Could you check a few things on this model? Use its own coordinates, in mm. Face numbers are marked on the shaded views. A direction names the side the tool comes from. Give positions to 0.01 mm unless a question says otherwise; leave off trailing zeros. Loops run counter-clockwise (first coordinate to the right, second up) from the corner with the lowest first, then second, coordinate; pieces in that order, holes last. Notation, with made-up numbers: (-10, -14) - (14, -14) arc R20 cw to (14, 13) - close; hole circle Ø1 at (76.25, -3.5). An arc over 180 degrees is marked (long way). Answer in a Markdown table with one row per item. Add a question column.
```python
from build123d import *

# Parameters (mm, degrees)
SKETCH_2_W          = 56
SKETCH_2_H          = 30
EXTRUDE_2_DEPTH     = 12
CUT_EXTRUDE_1_DEPTH = 65.652919501
SKETCH_6_W          = 24
SKETCH_6_H          = 30
CUT_EXTRUDE_2_DEPTH = 4
SKETCH_8_W          = 10
SKETCH_8_H          = 8
EXTRUDE_1_DEPTH     = 8
SKETCH_9_W          = 24
SKETCH_9_H          = 12
EXTRUDE_3_DEPTH     = 13
SKETCH_10_R         = 12
EXTRUDE_4_DEPTH     = 12
EXTRUDE_START       = -8
EXTRUDE_5_DEPTH     = 8
CUT_EXTRUDE_3_DEPTH = 68.446274916


with BuildPart() as part:
    # 草图2 → 凸台-拉伸2 (new body)
    with BuildSketch(Plane(origin=(0, 0, 0), x_dir=(1, 0, 0), z_dir=(0, 1, 0))):
        with Locations((28, -15)):
            Rectangle(SKETCH_2_W, SKETCH_2_H)
    extrude(amount=EXTRUDE_2_DEPTH)

    # 草图4 → 切除-拉伸1 (cut, through all)
    with BuildSketch(Plane.ZY):
        Polygon((9, 0), (21, 0), (23.886751346, 5), (6.113248654, 5), align=None)
    extrude(amount=-CUT_EXTRUDE_1_DEPTH, mode=Mode.SUBTRACT)

    # 草图6 → 切除-拉伸2 (cut)
    with BuildSketch(Plane(origin=(0, 12, 0), x_dir=(1, 0, 0), z_dir=(0, 1, 0))):
        with Locations((44, -15)):
            Rectangle(SKETCH_6_W, SKETCH_6_H)
    extrude(amount=-CUT_EXTRUDE_2_DEPTH, mode=Mode.SUBTRACT)

    # 草图8 → 拉伸-薄壁1 (add)
    with BuildSketch(Plane(origin=(0, 12, 0), x_dir=(1, 0, 0), z_dir=(0, 1, 0))):
        with Locations((5, -4)):
            Rectangle(SKETCH_8_W, SKETCH_8_H)
    extrude(amount=EXTRUDE_1_DEPTH)

    # 草图9 → 凸台-拉伸3 (add)
    with BuildSketch(Plane(origin=(0, 8, 0), x_dir=(1, 0, 0), z_dir=(0, 1, 0))):
        with Locations((44, -6)):
            Rectangle(SKETCH_9_W, SKETCH_9_H)
    extrude(amount=EXTRUDE_3_DEPTH)

    # 草图10 → 凸台-拉伸4 (add)
    with BuildSketch(Plane.XY.offset(12)):
        with Locations((44, 21)):
            Circle(SKETCH_10_R)
    extrude(amount=-EXTRUDE_4_DEPTH)

    # 草图13 → 凸台-拉伸5 (add)
    with BuildSketch(Plane(origin=(0, 0, 0), x_dir=(-1, 0, 0), z_dir=(0, 0, -1)).offset(EXTRUDE_START)):
        with BuildLine():
            Line((0, 20), (-44, 33))
            ThreePointArc((-44, 33), (-44.170266358, 32.998791996), (-44.340498436, 32.995168228))
            Line((-44.340498436, 32.995168228), (-44, 10))
            Line((-44, 10), (0, 10))
            Line((0, 10), (0, 20))
        make_face()
    extrude(amount=EXTRUDE_5_DEPTH)

    # 草图14 → 切除-拉伸3 (cut, through all)
    with BuildSketch(Plane.XY.offset(12)):
        with BuildLine():
            Line((38, 21), (38, 16))
            ThreePointArc((38, 16), (44, 10), (50, 16))
            Line((50, 16), (50, 21))
            ThreePointArc((50, 21), (44, 27), (38, 21))
        make_face()
    extrude(amount=-CUT_EXTRUDE_3_DEPTH, mode=Mode.SUBTRACT)


solid = part.part
```
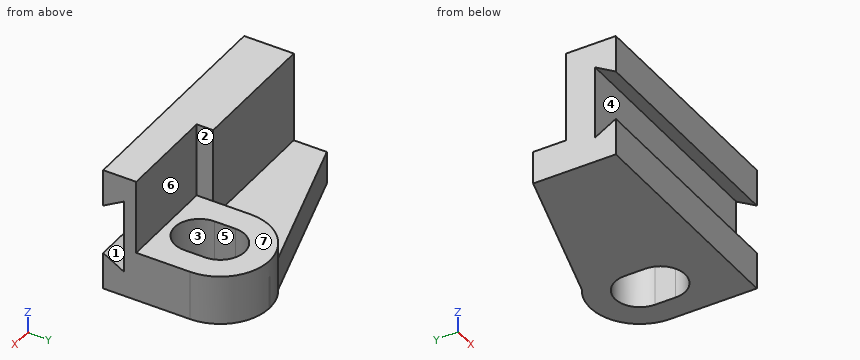
(1) I want a section at D-D on z = 22.5. Please give me the cut outline in (x, y), then the cut area to 3 significant figures.
(2) On a 3-axis mill with a long thin cutter (end or side, diameter ignored), from which of +Z, -Z, +X, -X, +Y, -Y can I reach the whole of each face in a straight line? I mean the marked faces 1, 2 and 3. Say none if no direction works.
(3) We'd pull the mould along Y, two halves only. Please class the marked faces 4, 5, 6 and 7: pulls with the +Y half, pulls with the -Y half, needs draft (parallel to the pull), parting line crosses it, or undercut.
(4) I want a section at B-B on y = 3. Please give me the cut outline in (x, z).
(5) I want a section at A-A on z = 25.5. Please give me the cut outline in (x, y), then the cut area to 3 significant figures.
(6) Please list where these lines run through material, in increasing order: line 1 (Y direction, x = 44, z = 7); line 2 (Y direction, x = 47, z = 14.25); line 3 (Y direction, x = 3.5, z = 27).
(7) For pin 1 Ø5.5 at (x, y) = (10.5, 21.5) entering from +Z; pin 2 Ø1.2 at (y, z) = (9.5, 22.5) entering from +X; pin 3 Ø1 at (x, z) = (28, 25.5) entering from +Y, each with a flat end and sliding along its axis, tell me the tip position at first contact or that it passes through.
(8) I want a section at C-C on x = 8. Please give me the cut outline in (y, z).
Reported:
| question | item | result |
|---|---|---|
| 1 | outline | (0, 0) - (56, 0) - (56, 2.6) - (0, 2.6) - close; (0, 5) - (56, 5) - (56, 8) - (32, 8) - (32, 12) - (0, 12) - close |
| 1 | area | 441 mm² |
| 2 | face 1 | +X, -X |
| 2 | face 2 | +Z, +X, +Y |
| 2 | face 3 | +Z, -Z |
| 3 | face 4 | undercut |
| 3 | face 5 | undercut |
| 3 | face 6 | pulls with the +Y half |
| 3 | face 7 | needs draft |
| 4 | outline | (0, 0) - (56, 0) - (56, 7.27) - (0, 7.27) - close; (0, 22.73) - (56, 22.73) - (56, 30) - (0, 30) - close |
| 5 | outline | (0, 0) - (56, 0) - (56, 8) - (32, 8) - (32, 12) - (0, 12) - close |
| 5 | area | 576 mm² |
| 6 | line 1 | 0 to 3.46, 5 to 10, 27 to 33 |
| 6 | line 2 | 5 to 8 |
| 6 | line 3 | 0 to 12 |
| 7 | pin 1 | z = 8 |
| 7 | pin 2 | x = 32 |
| 7 | pin 3 | y = 12 |
| 8 | outline | (0, 0) - (22.36, 0) - (22.36, 8) - (12, 8) - (12, 30) - (0, 30) - (0, 21) - (5, 23.89) - (5, 6.11) - (0, 9) - close |
